Geometry: final body of the model. Coordinates: model frame, mm. Face numbers are marked on the shaded views. A direction names the side the tool comes from. Give positions to 0.01 mm unless a question says otherwise; leave off trailing zeros. Write each loop counter-clockwise with the first axis right and the second up, starting at its lowest first coordinate (ties: lowest second). Pieces come first, ordered by that corner, then holes. Notation, with made-up numbers: (75, -35) -> (113, -35) arc R13 ccw to (113, -31) -> close; hole circle Ø1 at (-18.75, 88). An arc over 180 degrees is marked (long way). Answer in a Markdown table with one row per item. Add a question column.
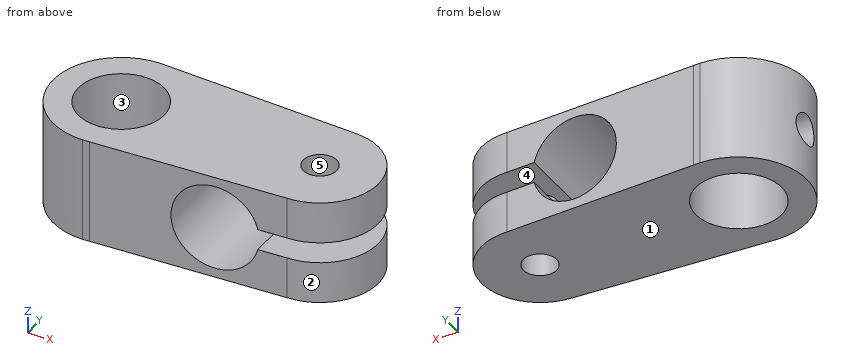
from build123d import *

# Parameters (mm, degrees)
SKETCH_1_R          = 4.1
EXTRUDE_1_DEPTH     = 10
SKETCH_6_R          = 4.1
CUT_EXTRUDE_2_DEPTH = 9.5
SKETCH_10_W         = 17.049616116
SKETCH_10_H         = 20.362574698
CUT_EXTRUDE_4_DEPTH = 1
SKETCH_11_R         = 1.6
CUT_EXTRUDE_5_DEPTH = 19.5
SKETCH_12_R         = 1.5
CUT_EXTRUDE_6_DEPTH = 39


with BuildPart() as part:
    # 草图1 → 凸台-拉伸1 (new body)
    with BuildSketch(Plane.XY):
        with BuildLine():
            Line((0.635580845, 6.468851288), (0, 6.5))
            ThreePointArc((0, 6.5), (-6.5, 0), (0, -6.5))
            Line((0, -6.5), (0.635580845, -6.468851288))
            Line((0.635580845, -6.468851288), (19, -5.568843046))
            ThreePointArc((19, -5.568843046), (24.568843046, 0), (19, 5.568843046))
            Line((19, 5.568843046), (0.635580845, 6.468851288))
        make_face()
        Circle(SKETCH_1_R, mode=Mode.SUBTRACT)
    extrude(amount=EXTRUDE_1_DEPTH)

    # 草图6 → 切除-拉伸2 (cut, symmetric)
    with BuildSketch(Plane(origin=(0, 0, 0), x_dir=(1, 0, 0), z_dir=(0, 1, 0))):
        with Locations((12.329939964, -5)):
            Circle(SKETCH_6_R)
    extrude(amount=CUT_EXTRUDE_2_DEPTH, both=True, mode=Mode.SUBTRACT)

    # 草图10 → 切除-拉伸4 (cut, symmetric)
    with BuildSketch(Plane.XY.offset(5)):
        with Locations((20.789235985, -0.838548644)):
            Rectangle(SKETCH_10_W, SKETCH_10_H)
    extrude(amount=CUT_EXTRUDE_4_DEPTH, both=True, mode=Mode.SUBTRACT)

    # 草图11 → 切除-拉伸5 (cut, symmetric)
    with BuildSketch(Plane.XY.offset(10)):
        with Locations((19, 0)):
            Circle(SKETCH_11_R)
    extrude(amount=CUT_EXTRUDE_5_DEPTH, both=True, mode=Mode.SUBTRACT)

    # 草图12 → 切除-拉伸6 (cut)
    with BuildSketch(Plane(origin=(0, 0, 0), x_dir=(0, 0, -1), z_dir=(1, 0, 0))):
        with Locations((-5, 0)):
            Circle(SKETCH_12_R)
    extrude(amount=-CUT_EXTRUDE_6_DEPTH, mode=Mode.SUBTRACT)


solid = part.part
Q1. Line query: probe 1 along Z at (x, y) = (-4.35, 0); probe 2 along X at (y, z) = (1.75, 7.5); probe 3 along X at (y, z) = (-2.5, 8.5). Output: solid intervals per line, ascending. Write a range as from..to.
Q2. Contact query for flat-ended pins moving along their axis: pin 1 Ø6.5 at (x, y) = (20, 0) entering from -Z; pin 2 Ø1.5 at (y, z) = (1.5, 2) entering from -X; pin 3 Ø5 at (x, z) = (20, 2.5) entering from -Y; pin 4 Ø4 at (x, z) = (8, 6) entering from -Y. Output: stop coordinate, or through.
Q3. Section D-D on z = 7.5. Return loops of the section in (x, y).
Q4. Section A-A on z = 2.25. Return loops of the section in (x, y).
Q5. Section C-C on x = 21. Return loops of the section in (y, z).
Q6. Pull-direction query (X, two-part tool) for the marked faces 1, 2 and 3; classes: +X half, -X half, draft (parallel to the pull), parting line (faces both ways), or undercut.
Q7. Section B-B on y = 0. Return loops of the section in (x, z), and give its area (3 significant figures).
Q8. Access query for the marked faces 4 and 5. Directions: +Z, -Z, +X, -X, +Y, -Y. A direction counts if a zero-diameter tool reaches every point of the face in a straight line with its end or side. Return the directions, or none.
Checks:
| question | item | result |
|---|---|---|
| 1 | probe 1 | 0..3.5, 6.5..10 |
| 1 | probe 2 | -6.26..-3.71, 3.71..9.08, 15.58..24.29 |
| 1 | probe 3 | -6..-3.25, 3.25..10.19, 14.47..23.98 |
| 2 | pin 1 | z = 0 |
| 2 | pin 2 | x = -6.46 |
| 2 | pin 3 | y = -5.64 |
| 2 | pin 4 | y = -6.21 |
| 3 | outline | (0, -6.5) -> (9.08, -6.05) -> (9.08, 6.05) -> (0, 6.5) arc R6.5 ccw to start; (15.58, -5.74) -> (19, -5.57) arc R5.57 ccw to (19, 5.57) -> (15.58, 5.74) -> close; hole circle Ø8.2 at (0, 0); hole circle Ø3.2 at (19, 0) |
| 4 | outline | (0, -6.5) -> (9.29, -6.04) -> (9.29, 6.04) -> (0, 6.5) arc R6.5 ccw to start; (15.37, -5.75) -> (19, -5.57) arc R5.57 ccw to (19, 5.57) -> (15.37, 5.75) -> close; hole circle Ø8.2 at (0, 0); hole circle Ø3.2 at (19, 0) |
| 5 | outline | (-5.2, 0) -> (5.2, 0) -> (5.2, 4) -> (-5.2, 4) -> close; (-5.2, 6) -> (5.2, 6) -> (5.2, 10) -> (-5.2, 10) -> close |
| 6 | face 1 | draft |
| 6 | face 2 | +X half |
| 6 | face 3 | undercut |
| 7 | outline | (-6.5, 0) -> (-4.1, 0) -> (-4.1, 3.5) -> (-6.5, 3.5) -> close; (-6.5, 6.5) -> (-4.1, 6.5) -> (-4.1, 10) -> (-6.5, 10) -> close; (4.1, 0) -> (17.4, 0) -> (17.4, 4) -> (16.31, 4) arc R4.1 cw (long way) to (16.31, 6) -> (17.4, 6) -> (17.4, 10) -> (4.1, 10) -> close; (20.6, 0) -> (24.57, 0) -> (24.57, 4) -> (20.6, 4) -> close; (20.6, 6) -> (24.57, 6) -> (24.57, 10) -> (20.6, 10) -> close |
| 7 | area | 127 mm^2 |
| 8 | face 4 | +X, +Y, -Y |
| 8 | face 5 | +Z, -Z |
